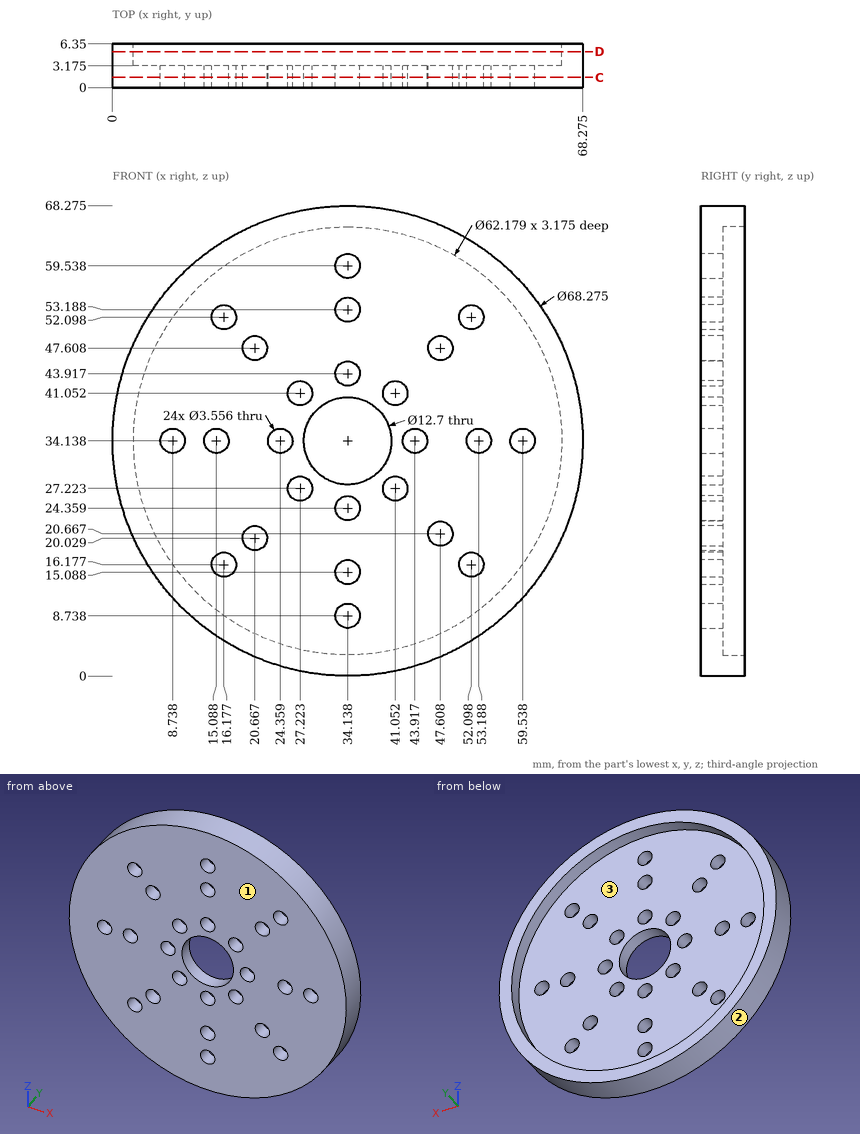
Design review of the part shown in the three views and the two pictorial views. Dimensions are in mm from the part's minimum x, y and z. Round coordinates to 2 decimals unless told otherwise and drop trailing zeros. Write each loop counter-clockwise with the first axis right and the second up, starting at its lowest first coordinate (ties: lowest second). Pieces come first, ordered by that corner, then holes.
Item 1: We need section D-D on y = 5.25. Write out the cut boundary in (x, z) (1 decimal).
Item 2: Clearance check with flat-ended pins moving along their axes: pin 1 Ø3 at (x, y) = (38.5, 1) entering from -Z; pin 2 Ø4 at (x, z) = (47.61, 20.67) entering from +Y (3 decimals). State where each tip first meets the part, or that it passes through.
Item 3: For probe 1 along X at (y, z) = (2, 15) (1 decimal); probe 2 along X at (y, z) = (1, 40) (1 decimal); probe 3 along X at (y, z) = (4.75, 51) (1 decimal), list the stretches that pass through material, from the lowest coordinate up.
Item 4: The part is to be moulded in two halves that separate along X. For the marked faces 1, 2 and 3, say which applies: +X half, -X half, draft (parallel to the pull), parting line (faces both ways), or undercut.
Item 5: We need section C-C on y = 1.5. State how many separate pieces and enclosed holes the cut face has, and give its area (3 significant figures).
Returned:
1. outline: circle Ø68.3 at (34.1, 34.1); hole circle Ø62.2 at (34.1, 34.1)
2. pin 1: stops at z = 0.12
2. pin 2: stops at y = 3.175
3. probe 1: x = 5.9 to 14.8, 17.5 to 32.4, 35.9 to 50.8, 53.4 to 62.4
3. probe 2: x = 0.5 to 25.8, 28.7 to 31.7, 36.6 to 39.6, 42.5 to 67.8
3. probe 3: x = 4.5 to 8, 60.3 to 63.8
4. face 1: draft
4. face 2: parting line
4. face 3: undercut
5. separate pieces: 1
5. enclosed holes: 25
5. area: 3,300 mm2
